from build123d import *

# Parameters (mm, degrees)
F0_R     = 11.175
F0_R_2   = 10
F0_R_3   = 3.9
F0_R_4   = 2.5
F1_DEPTH = 1
F2_DEPTH = 7
F3_DEPTH = 3.5


with BuildPart() as f1:
    # F0 (on Top) → F1 (new body)
    with BuildSketch(Plane.XY):
        with BuildLine():
            ThreePointArc((11.4011948308, -9.7474487139), (14.0715656993, -5.1952900563), (15, 0))
            ThreePointArc((15, 0), (14.0715656993, 5.1952900563), (11.4011948308, 9.7474487139))
            ThreePointArc((11.4011948308, 9.7474487139), (7.5, 12.9903810568), (2.7409407929, 14.7474487139))
            ThreePointArc((2.7409407929, 14.7474487139), (-7.5, 12.9903810568), (-14.1421356237, 5))
            ThreePointArc((-14.1421356237, 5), (-15, 0), (-14.1421356237, -5))
            ThreePointArc((-14.1421356237, -5), (-7.5, -12.9903810568), (2.7409407929, -14.7474487139))
            ThreePointArc((2.7409407929, -14.7474487139), (7.5, -12.9903810568), (11.4011948308, -9.7474487139))
        make_face()
        Circle(F0_R, mode=Mode.SUBTRACT)
        Circle(F0_R)
        Circle(F0_R_2, mode=Mode.SUBTRACT)
        with BuildLine():
            ThreePointArc((-14.1421356237, -5), (-15, 0), (-14.1421356237, 5))
            ThreePointArc((-14.1421356237, 5), (-22.0710678119, 7.2668921957), (-30, 5))
            ThreePointArc((-30, 5), (-26.4644660941, 3.5355339059), (-25, 0))
            ThreePointArc((-25, 0), (-25.3292685703, -1.7844517118), (-26.2737071647, -3.333877878))
            ThreePointArc((-26.2737071647, -3.333877878), (-20.0301598509, -2.8725999161), (-14.1421356237, -5))
        make_face()
        with BuildLine():
            ThreePointArc((2.7409407929, 14.7474487139), (7.5, 12.9903810568), (11.4011948308, 9.7474487139))
            ThreePointArc((11.4011948308, 9.7474487139), (17.328847154, 15.4806593159), (19.3301270189, 23.4807621135))
            ThreePointArc((19.3301270189, 23.4807621135), (14.4852262544, 21.0073319099), (10.2496306469, 24.4206367952))
            ThreePointArc((10.2496306469, 24.4206367952), (7.5273354232, 18.7829272308), (2.7409407929, 14.7474487139))
        make_face()
        with BuildLine():
            ThreePointArc((16.0240765178, -21.0867589172), (12.5028244277, -15.9103273147), (11.4011948308, -9.7474487139))
            ThreePointArc((11.4011948308, -9.7474487139), (7.5, -12.9903810568), (2.7409407929, -14.7474487139))
            ThreePointArc((2.7409407929, -14.7474487139), (4.7422206579, -22.7475515116), (10.6698729811, -28.4807621135))
            ThreePointArc((10.6698729811, -28.4807621135), (10.9502699725, -23.0482398708), (16.0240765178, -21.0867589172))
        make_face()
        with BuildLine():
            ThreePointArc((-25, 0), (-26.4644660941, 3.5355339059), (-30, 5))
            ThreePointArc((-30, 5), (-35, 0), (-30, -5))
            ThreePointArc((-30, -5), (-28.1937916946, -4.0395964849), (-26.2737071647, -3.333877878))
            ThreePointArc((-26.2737071647, -3.333877878), (-25.3292685703, -1.7844517118), (-25, 0))
        make_face()
        with Locations((-30, 0)):
            Circle(F0_R_3, mode=Mode.SUBTRACT)
        with BuildLine():
            ThreePointArc((19.3301270189, -23.4807621135), (17.5952890243, -22.3967415941), (16.0240765178, -21.0867589172))
            ThreePointArc((16.0240765178, -21.0867589172), (10.9502699725, -23.0482398708), (10.6698729811, -28.4807621135))
            ThreePointArc((10.6698729811, -28.4807621135), (16.2940952255, -30.810391245), (20, -25.9807621135))
            ThreePointArc((20, -25.9807621135), (19.8296291314, -24.686666888), (19.3301270189, -23.4807621135))
        make_face()
        with Locations((15, -25.9807621135)):
            Circle(F0_R_3, mode=Mode.SUBTRACT)
        with BuildLine():
            ThreePointArc((10.2496306469, 24.4206367952), (14.4852262544, 21.0073319099), (19.3301270189, 23.4807621135))
            ThreePointArc((19.3301270189, 23.4807621135), (19.8296291314, 24.686666888), (20, 25.9807621135))
            ThreePointArc((20, 25.9807621135), (16.2940952255, 30.810391245), (10.6698729811, 28.4807621135))
            ThreePointArc((10.6698729811, 28.4807621135), (10.5985026704, 26.436338079), (10.2496306469, 24.4206367952))
        make_face()
        with Locations((15, 25.9807621135)):
            Circle(F0_R_3, mode=Mode.SUBTRACT)
        with Locations((-30, 0)):
            Circle(F0_R_3)
        with Locations((-30, 0)):
            Circle(F0_R_4, mode=Mode.SUBTRACT)
        with Locations((15, -25.9807621135)):
            Circle(F0_R_3)
        with Locations((15, -25.9807621135)):
            Circle(F0_R_4, mode=Mode.SUBTRACT)
        with Locations((15, 25.9807621135)):
            Circle(F0_R_3)
        with Locations((15, 25.9807621135)):
            Circle(F0_R_4, mode=Mode.SUBTRACT)
        with Locations((-30, 0)):
            Circle(F0_R_4)
        with Locations((15, -25.9807621135)):
            Circle(F0_R_4)
        with Locations((15, 25.9807621135)):
            Circle(F0_R_4)
        with BuildLine():
            ThreePointArc((-30, -5), (-27.9590920391, -4.5645037731), (-26.2737071647, -3.333877878))
            ThreePointArc((-26.2737071647, -3.333877878), (-28.1937916946, -4.0395964849), (-30, -5))
        make_face()
        with BuildLine():
            ThreePointArc((19.3301270189, -23.4807621135), (17.9325222427, -21.931032086), (16.0240765178, -21.0867589172))
            ThreePointArc((16.0240765178, -21.0867589172), (17.5952890243, -22.3967415941), (19.3301270189, -23.4807621135))
        make_face()
        with BuildLine():
            ThreePointArc((10.6698729811, 28.4807621135), (10.0265697963, 26.4955358592), (10.2496306469, 24.4206367952))
            ThreePointArc((10.2496306469, 24.4206367952), (10.5985026704, 26.436338079), (10.6698729811, 28.4807621135))
        make_face()
    extrude(amount=-F1_DEPTH)

    # F0 (on Top) → F2 (join)
    with BuildSketch(Plane.XY):
        with Locations((-30, 0)):
            Circle(F0_R_3)
        with Locations((-30, 0)):
            Circle(F0_R_4, mode=Mode.SUBTRACT)
        with Locations((15, 25.9807621135)):
            Circle(F0_R_3)
        with Locations((15, 25.9807621135)):
            Circle(F0_R_4, mode=Mode.SUBTRACT)
        with Locations((15, -25.9807621135)):
            Circle(F0_R_3)
        with Locations((15, -25.9807621135)):
            Circle(F0_R_4, mode=Mode.SUBTRACT)
    extrude(amount=F2_DEPTH)

    # F0 (on Top) → F3 (join)
    with BuildSketch(Plane.XY):
        with BuildLine():
            ThreePointArc((11.4011948308, -9.7474487139), (14.0715656993, -5.1952900563), (15, 0))
            ThreePointArc((15, 0), (14.0715656993, 5.1952900563), (11.4011948308, 9.7474487139))
            ThreePointArc((11.4011948308, 9.7474487139), (7.5, 12.9903810568), (2.7409407929, 14.7474487139))
            ThreePointArc((2.7409407929, 14.7474487139), (-7.5, 12.9903810568), (-14.1421356237, 5))
            ThreePointArc((-14.1421356237, 5), (-15, 0), (-14.1421356237, -5))
            ThreePointArc((-14.1421356237, -5), (-7.5, -12.9903810568), (2.7409407929, -14.7474487139))
            ThreePointArc((2.7409407929, -14.7474487139), (7.5, -12.9903810568), (11.4011948308, -9.7474487139))
        make_face()
        Circle(F0_R, mode=Mode.SUBTRACT)
    extrude(amount=F3_DEPTH)


solid = f1.part
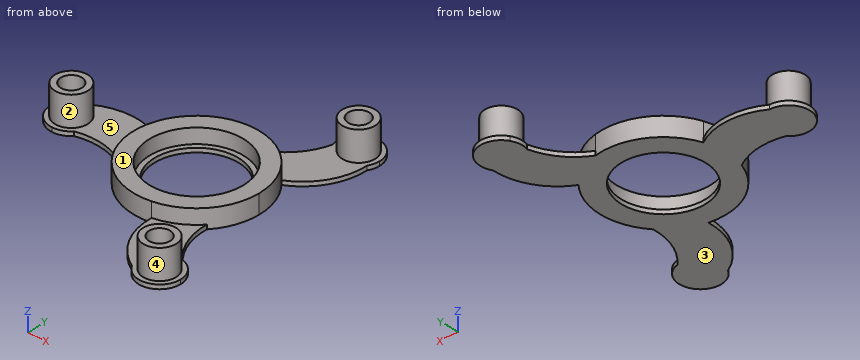
The model under review builds one solid part; all positions refer to its coordinate system, in mm. Face numbers are marked on the shaded views. A direction names the side the tool comes from. Give positions to 0.01 mm unless a question says otherwise; leave off trailing zeros. Order: outer loops, then holes, each group sorted by start corner. A loop starts at its lowest first (then second) coordinate and runs counter-clockwise, first axis right, second up. Notation, with made-up numbers: M 18.25,75 L 70.25,75 A13 ccw 70.25,90 Z; hole C 63,21 d2. An arc over 180 degrees is marked long. Answer in a Markdown table with one row per item. Add a question column.
1. Add section B-B on z = 6. State the section outline as (x, y) points.
2. Mouldability with a two-part tool opening along X and no side actions: class the marked faces 3, 4 and 5 as released by +X, released by -X, zero draft, split by the parting line, or undercut.
3. Add section C-C on x = -1. State the section outline as (y, z) points, plus the area to 3 significant figures.
4. For pin 1 Ø5 at (x, y) = (12, -16.5) entering from +Z; pin 2 Ø15 at (x, y) = (-5, -0.5) entering from +Z; pin 3 Ø4 at (y, z) = (-6, 0.5) entering from -X, all flat-tipped, find the tip position at first contact; note any pin that passes through.
5. To check wall thickness, follow line 1 along Y through (x, z) = (15, 3.5); line 2 along Y through (x, z) = (-30, 3.75); line 3 along Y through (x, z) = (0, -0.25). State the ranges of each line that lie inside material, in increasing order.
6. Add section D-D on y = -1. State the section outline as (x, z) points, plus the area to 3 significant figures.
7. Add section A-A on z = 2.5. State the section outline as (x, y) points (3 decimals).
8. Machinability: for the marked faces 1 and 2, which of the approach directions +Z, -Z, +X, -X, +Y, -Y give a long, thin tool a straight path to every point of the face, cutting with its end or side? Answer none if there is none.
The answers:
| question | item | result |
|---|---|---|
| 1 | outline | C -30,0 d7.8; C 15,-25.98 d7.8; C 15,25.98 d7.8; hole C -30,0 d5; hole C 15,-25.98 d5; hole C 15,25.98 d5 |
| 2 | face 3 | zero draft |
| 2 | face 4 | split by the parting line |
| 2 | face 5 | undercut |
| 3 | outline | M -14.97,-1 L -9.95,-1 L -9.95,0 L -11.13,0 L -11.13,3.5 L -14.97,3.5 Z; M 9.95,-1 L 14.97,-1 L 14.97,3.5 L 11.13,3.5 L 11.13,0 L 9.95,0 Z |
| 3 | area | 36.9 mm2 |
| 4 | pin 1 | z = 0 |
| 4 | pin 2 | z = 3.5 |
| 4 | pin 3 | x = -32.91 |
| 5 | line 1 | -29.88 to -28.48, -23.48 to -22.08, 22.08 to 23.48, 28.48 to 29.88 |
| 5 | line 2 | -3.9 to -2.5, 2.5 to 3.9 |
| 5 | line 3 | -15 to -10, 10 to 15 |
| 6 | outline | M -34.9,-1 L -9.95,-1 L -9.95,0 L -11.13,0 L -11.13,3.5 L -14.97,3.5 L -14.97,0 L -26.23,0 L -26.23,7 L -27.71,7 L -27.71,0 L -32.29,0 L -32.29,7 L -33.77,7 L -33.77,0 L -34.9,0 Z; M 9.95,-1 L 14.97,-1 L 14.97,3.5 L 11.13,3.5 L 11.13,0 L 9.95,0 Z |
| 6 | area | 77.5 mm2 |
| 7 | outline | C -30,0 d7.8; C 0,0 d30; C 15,-25.981 d7.8; C 15,25.981 d7.8; hole C -30,0 d5; hole C 0,0 d22.35; hole C 15,-25.981 d5; hole C 15,25.981 d5 |
| 8 | face 1 | +Z, +X |
| 8 | face 2 | +Z |
